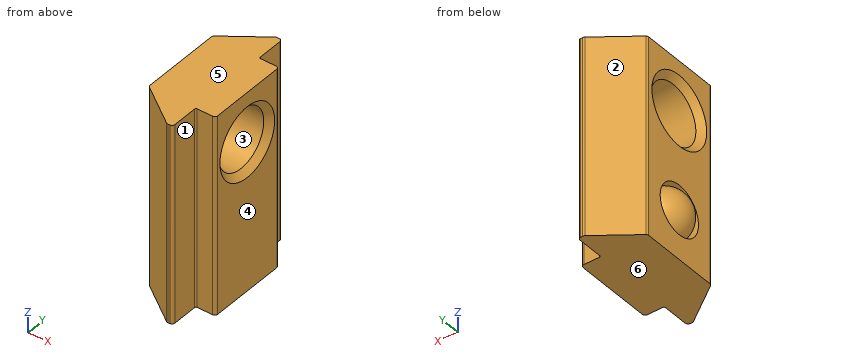
Autodesk Inventor part; units mm, degrees
ref_plane "to_blackets_XY" through (0, 0, -3.5) normal (1, 0, 0) x (0, 0, -1)
ref_plane "to_blackets_YZ" through (0, 0, -3.5) normal (0, 0, -1) x (0, 1, 0)
ref_plane "to_blackets_ZX" through (0, 0, -3.5) normal (0, 1, 0) x (1, 0, 0)
sketch "_____1" plane through (0, 0, 0) normal (0, 0, 1) x (1, 0, 0)
  line L0 (-4.7, 2.7981) -> (-4.7, -2.7981)
  arc A0 (-4.7, -2.7981) -> (-4.6176, -2.9599) centre (-4.5, -2.7981) ccw
  line L1 (-4.6176, -2.9599) -> (-1.8622, -4.9618)
  arc A1 (-1.8622, -4.9618) -> (-1.7446, -5) centre (-1.7446, -4.8) ccw
  line L2 (-1.7446, -5) -> (-1.6, -5)
  arc A2 (-1.6, -5) -> (-1.4, -4.8) centre (-1.6, -4.8) ccw
  line L3 (-1.4, -4.8) -> (-1.4, -3)
  arc A3 (-1.3, -2.9) -> (-1.4, -3) centre (-1.3, -3) ccw
  line L4 (-1.3, -2.9) -> (-0.2, -2.9)
  arc A4 (-0.2, -2.9) -> (0, -2.7) centre (-0.2, -2.7) ccw
  line L5 (0, -2.7) -> (0, 2.7)
  arc A5 (0, 2.7) -> (-0.2, 2.9) centre (-0.2, 2.7) ccw
  line L6 (-0.2, 2.9) -> (-1.3, 2.9)
  arc A6 (-1.4, 3) -> (-1.3, 2.9) centre (-1.3, 3) ccw
  line L7 (-1.4, 3) -> (-1.4, 4.8)
  arc A7 (-1.4, 4.8) -> (-1.6, 5) centre (-1.6, 4.8) ccw
  line L8 (-1.6, 5) -> (-1.7446, 5)
  arc A8 (-1.7446, 5) -> (-1.8622, 4.9618) centre (-1.7446, 4.8) ccw
  line L9 (-1.8622, 4.9618) -> (-4.6176, 2.9599)
  arc A9 (-4.6176, 2.9599) -> (-4.7, 2.7981) centre (-4.5, 2.7981) ccw
extrude "Extrusion1" add sketch "_____1" against normal blind 14
sketch "_____2" plane through (0, 0, -3.5) normal (0, 0, 1) x (1, 0, 0)
  line L0 (0, 0) -> (-4.7, 0)
  line L1 (-4.7, 0) -> (-4.7, 2.5)
  line L2 (-4.7, 2.5) -> (-4.267, 2.067)
  line L3 (-4.267, 2.067) -> (-0.433, 2.067)
  line L4 (-0.433, 2.067) -> (0, 2.5)
  line L5 (0, 2.5) -> (0, 0)
  line L6 (0, 0) -> (-4.7, 0)
revolve "Revolution1" cut sketch "_____2" angle 360 about axis through (0, 0, -3.5) along (1, 0, 0)
thread "Thread1"
sketch "_____3" plane through (0, 0, -10.5) normal (0, 0, 1) x (1, 0, 0)
  line L0 (-3.65, 0) -> (-5.4, 0)
  line L1 (-5.4, 0) -> (-5.4, 1.75)
  line L2 (-5.4, 1.75) -> (-3.65, 1.75)
  line L3 (-3.65, 1.75) -> (-3.65, 0)
  line L4 (-3.65, 0) -> (-5.4, 0)
revolve "Revolution2" cut sketch "_____3" angle 360 about axis through (-3.65, 0, -10.5) along (1, 0, 0)
sketch "_____4" plane through (0, 0, -10.5) normal (0, 0, 1) x (1, 0, 0)
  line L0 (-3.65, 1.75) -> (-3.65, -1.75)
  arc A0 (-3.65, 1.75) -> (-3.65, -1.75) centre (-3.65, 0) ccw
  line L1 (-3.65, 1.75) -> (-3.65, -1.75)
revolve "Revolution3" add sketch "_____4" angle 360 about axis through (-3.65, 1.75, -10.5) along (0, 1, 0)
ref_plane "to_blackets_XY" through (0, 0, -3.5) normal (1, 0, 0) x (0, 0, -1)
ref_plane "to_blackets_YZ" through (0, 0, -3.5) normal (0, 0, -1) x (0, 1, 0)
ref_plane "to_blackets_ZX" through (0, 0, -3.5) normal (0, 1, 0) x (1, 0, 0)
ref_plane "to_bolt_XY" through (-4.7, 0, -3.5) normal (1, 0, 0) x (0, 0, -1)
ref_plane "to_bolt_YZ" through (-4.7, 0, -3.5) normal (0, 0, -1) x (0, 1, 0)
ref_plane "to_bolt_ZX" through (-4.7, 0, -3.5) normal (0, 1, 0) x (1, 0, 0)
ref_plane "to_frames_XY" through (-1.4, 0, -3.5) normal (1, 0, 0) x (0, 0, -1)
ref_plane "to_frames_YZ" through (-1.4, 0, -3.5) normal (0, 0, -1) x (0, 1, 0)
ref_plane "to_frames_ZX" through (-1.4, 0, -3.5) normal (0, 1, 0) x (1, 0, 0)
properties part number "SHNTU5-5"
Read the model definition and answer for the solid it produces. Units are mm, in the model's axes. Face numbers are marked on the shaded views. A direction names the side the tool comes from. Coordinates: 2 decimals unless noted, no trailing zeros. Write each loop counter-clockwise with the first axis right and the second up, starting at its lowest first coordinate (ties: lowest second). Pieces come first, ordered by that corner, then holes. Notation, with made-up numbers: (44.25, 51) - (94.25, 51) arc R35 ccw to (94.25, 87) - close; hole circle Ø2 at (72.25, 46). An arc over 180 degrees is marked (long way). One line per question, with ' | ' between items.
Q1. Consider L1, parallel to Z at x = -1.3, y = 0; L2, parallel to X at y = -2.25, z = -10; L3, parallel to Y at x = -0.35, z = -2.5. Determine where each line is inside the solid, lowest interval first. Write a range as [from, to].
Result set:
L1: [-14, -5.57], [-1.43, 0] | L2: [-4.7, 0] | L3: [-2.9, -1.9], [1.9, 2.9]
Q2. Find section B-B, the plane x = -3.85. Write down the section's boundary in (y, z).
Result set:
outline: (-3.52, -14) - (3.52, -14) - (3.52, 0) - (-3.52, 0) - close; circle Ø3.48 at (0, -10.5); hole circle Ø4.13 at (0, -3.5); hole circle Ø3.5 at (0, -10.5)
Q3. For the marked faces 1 and 2, determine the directions among +Z, -Z, +X, -X, +Y, -Y from which every point of the face is accessible in a straight line to the end or side of a thin tool.
Result set:
face 1: +Z, -Z, +X, -Y | face 2: +Z, -Z, -X, +Y
Q4. Determine the mould class of the marked faces 3, 4, 5 and 6 for opening direction Z: +Z half, -Z half, draft (parallel to the pull), parting line (faces both ways), or undercut.
Result set:
face 3: undercut | face 4: draft | face 5: +Z half | face 6: -Z half
Q5. Find section D-D, the plane x = -0.75. Write down the section's boundary in (y, z), plus the area to 3 significant figures.
Result set:
outline: (-2.9, -14) - (2.9, -14) - (2.9, 0) - (-2.9, 0) - close; hole circle Ø4.13 at (0, -3.5) | area: 67.8 mm^2
Q6. Find section A-A, the plane z = -3.5. Write down the section's boundary in (x, y).
Result set:
outline: (-4.7, -2.8) arc R0.2 ccw to (-4.62, -2.96) - (-1.86, -4.96) arc R0.2 ccw to (-1.74, -5) - (-1.6, -5) arc R0.2 ccw to (-1.4, -4.8) - (-1.4, -3) arc R0.1 cw to (-1.3, -2.9) - (-0.2, -2.9) arc R0.2 ccw to (0, -2.7) - (0, -2.5) - (-0.43, -2.07) - (-4.27, -2.07) - (-4.7, -2.5) - close; (-4.7, 2.5) - (-4.27, 2.07) - (-0.43, 2.07) - (0, 2.5) - (0, 2.7) arc R0.2 ccw to (-0.2, 2.9) - (-1.3, 2.9) arc R0.1 cw to (-1.4, 3) - (-1.4, 4.8) arc R0.2 ccw to (-1.6, 5) - (-1.74, 5) arc R0.2 ccw to (-1.86, 4.96) - (-4.62, 2.96) arc R0.2 ccw to (-4.7, 2.8) - close
Q7. Each of these flat-tipped pins is pushed along its axis until it touches: P1, Ø3, axis at y = 3.5, z = -10, coming from the -X side; P2, Ø1.4, axis at y = -4, z = -7.5, coming from the +X side; P3, Ø0.6, axis at x = -1, z = -9.5, coming from the +Y side. Where does it stop, or does it pass through?
Result set:
P1: x = -4.7 | P2: x = -1.4 | P3: y = 2.9
Q8. Find section C-C, the plane y = 0. Write down the section's boundary in (x, z), plus the area to 3 significant figures.
Result set:
outline: (-4.7, -14) - (0, -14) - (0, -6) - (-0.43, -5.57) - (-4.27, -5.57) - (-4.7, -6) - (-4.7, -8.75) - (-3.65, -8.75) arc R1.75 ccw to (-3.65, -12.25) - (-4.7, -12.25) - close; (-4.7, -1) - (-4.27, -1.43) - (-0.43, -1.43) - (0, -1) - (0, 0) - (-4.7, 0) - close | area: 47.1 mm^2
